Here's how the part is built. I have some questions about the finished solid (model axes, mm). A direction names the side the tool comes from. Give positions to 0.01 mm unless a question says otherwise; leave off trailing zeros. Loops run counter-clockwise (first coordinate to the right, second up) from the corner with the lowest first, then second, coordinate; pieces in that order, holes last.
Q1. For faces 4 (the face through (29.964, 1.476, 1.29)), 5 (the face through (25, 0.8, 0.5)), which set-ups out of +Z, -Z, +X, -X, +Y, -Y let a thin tool reach every point of the face, with its end or its side?
Q2. Suppose I cut it at C-C (z = 0). List the corners of the cut face in (x, y) for me.
Q3. Suppose I cut it at B-B (y = 3.5). List the corners of the cut face in (x, z) for me, and give its area (3 significant figures).
Q4. I'm going to push a flat-ended pin straight in: P1, Ø23, axis at x = 5.5, z = 16.5, coming from the -Y side. Where does the tip first touch, or does it pass through?
Q5. Suppose I cut it at D-D (z = -24). List the corners of the cut face in (x, y) for me, and give its area (3 significant figures).
Q6. Suppose I cut it at A-A (x = 18). List the corners of the cut face in (y, z) for me.
Q7. I need wall thicknesses on probe 1 along Z at (x, y) = (28, 3.5); probe 2 along X at (y, z) = (7.8, -24); probe 3 along Z at (x, y) = (18, 9.2). Which ranges of each line are inside material? Lowest first, please.
Q8. Thinking about a two-plate mould opening in Z: for faces 1 (the face through (0.5, 7.2, 35)), 2 (the face through (-19.586, 8.479, -24.208)), 3 (the face through (-24.43, 6.4, -0.49)), which applies, pulls with the +Z half, pulls with the -Z half, needs draft (parallel to the pull), parting line crosses it, or undercut?
Autodesk Inventor part; units mm, degrees
ref_plane "YZ Plane" through (0, 0, 0) normal (1, 0, 0) x (0, 1, 0)
ref_plane "XZ Plane" through (0, 0, 0) normal (0, 1, 0) x (-1, 0, 0)
ref_plane "XY Plane" through (0, 0, 0) normal (0, 0, 1) x (1, 0, 0)
sketch "スケッチ1" plane through (0, 0, 0) normal (0, 1, 0) x (-1, 0, 0)
  line L0 (35, -35) -> (-35, -35)
  line L1 (-35, -35) -> (-35, 35)
  line L2 (-35, 35) -> (35, 35)
  line L3 (35, 35) -> (35, -35)
  line L4 (35, -35) -> (-35, 35) construction
  line L5 (-35, -35) -> (35, 35) construction
  point P0 (0, 0)
  dimension "d0" = 70
  dimension "d1" = 70
extrude "押し出し1" add sketch "スケッチ1" along normal blind 10
sketch "スケッチ2" plane through (0, 0, 0) normal (0, -1, 0) x (1, 0, 0)
  line L0 (35, -35) -> (-35, -35)
  line L1 (-25, 35) -> (25, 35)
  line L2 (25, 35) -> (25, -35)
  line L3 (25, -35) -> (-25, -35)
  line L4 (-25, -35) -> (-25, 35)
  line L5 (-25, 35) -> (25, -35) construction
  line L6 (25, 35) -> (-25, -35) construction
  point P0 (0, 0)
  dimension "d4" = 50
extrude "押し出し2" cut sketch "スケッチ2" against normal blind 7
sketch "スケッチ3" plane through (-35, 0, -35) normal (-1, 0, 0) x (0, 0, 1)
  line L0 (0, 0) -> (70, 0)
  point P0 (35, 0)
  point P1 (35, 3.5)
  point P2 (35, 0)
  dimension "d7" = 3.5
hole "穴1" at (-35, 3.5, 0) direction (1, 0, 0) diameter 4.8 end through all
sketch "スケッチ4" plane through (0, 10, 0) normal (0, 1, 0) x (1, 0, 0)
  line L0 (35, 35) -> (-35, 35)
  line L1 (-35, 35) -> (-35, -35)
  point P0 (0, 0)
  point P1 (-18, 24)
  point P2 (18, 24)
  point P3 (-18, -24)
  point P4 (18, -24)
  dimension "d15" = 18
  dimension "d16" = 24
  dimension "d17" = 11
  dimension "d18" = 17
  dimension "d21" = 36
  dimension "d24" = 48
hole "穴2" at (-18, 10, -24) at (18, 10, -24) at (-18, 10, 24) at (18, 10, 24) direction (0, -1, 0) diameter 3.2 end through all
sketch "スケッチ5" plane through (-35, 0, -35) normal (-1, 0, 0) x (0, 0, 1)
  line L0 (0, 0) -> (70, 0)
  circle A0 centre (35, 3.5) radius 2.4
  point P0 (35, 0)
  point P1 (65, 3.5)
  dimension "d34" = 3.5
  dimension "d35" = 30
hole "穴3" at (-35, 3.5, 30) direction (1, 0, 0) diameter 2.8 end through all
fillet "フィレット1" radius 2 6 edges at (-35, 5, 35) (-35, 5, -35) (35, 5, -35) (35, 5, 35) (25, 7, 0) (-25, 7, 0)
properties part number "MID-360_mountA"
Solutions:
1. face 4: +X, -X
1. face 5: +Z, -Z, -Y
2. outline: (-35, 0) - (-25, 0) - (-25, 1.1) - (-35, 1.1) - close; (-35, 5.9) - (-24.79, 5.9) arc R2 cw to (-23, 7) - (23, 7) arc R2 cw to (24.79, 5.9) - (35, 5.9) - (35, 10) - (-35, 10) - close; (25, 0) - (35, 0) - (35, 1.1) - (25, 1.1) - close
3. outline: (-35, -33) arc R2 ccw to (-33, -35) - (-25, -35) - (-25, -2.4) - (-35, -2.4) - close; (-35, 2.4) - (-25, 2.4) - (-25, 28.6) - (-35, 28.6) - close; (-35, 31.4) - (-25, 31.4) - (-25, 35) - (-33, 35) arc R2 ccw to (-35, 33) - close; (25, -35) - (33, -35) arc R2 ccw to (35, -33) - (35, -2.4) - (25, -2.4) - close; (25, 2.4) - (35, 2.4) - (35, 28.6) - (25, 28.6) - close; (25, 31.4) - (35, 31.4) - (35, 33) arc R2 ccw to (33, 35) - (25, 35) - close
3. area: 1,240 mm2
4. P1: stops at y = 7
5. outline: (-35, 0) - (-25, 0) - (-25, 5) arc R2 cw to (-23, 7) - (-19.6, 7) - (-19.6, 10) - (-35, 10) - close; (-16.4, 7) - (16.4, 7) - (16.4, 10) - (-16.4, 10) - close; (19.6, 7) - (23, 7) arc R2 cw to (25, 5) - (25, 0) - (35, 0) - (35, 10) - (19.6, 10) - close
5. area: 333 mm2
6. outline: (7, -35) - (10, -35) - (10, -25.6) - (7, -25.6) - close; (7, -22.4) - (10, -22.4) - (10, 22.4) - (7, 22.4) - close; (7, 25.6) - (10, 25.6) - (10, 35) - (7, 35) - close
7. probe 1: z = -35 to -2.4, 2.4 to 28.6, 31.4 to 35
7. probe 2: x = -35 to -19.6, -16.4 to 16.4, 19.6 to 35
7. probe 3: z = -35 to -25.6, -22.4 to 22.4, 25.6 to 35
8. face 1: pulls with the +Z half
8. face 2: undercut
8. face 3: needs draft
